Check sheet for the drawn part. Datum: minimum x, y, z corner. Units: mm. A direction names the side the tool comes from. Coordinates: 2 decimals unless noted, no trailing zeros. Write each loop counter-clockwise with the first axis right and the second up, starting at its lowest first coordinate (ties: lowest second). Pieces come first, ordered by that corner, then holes. Notation, with made-up numbers: M 58,-32.5 L 87,-32.5 A23 cw 87,-4.5 Z; hole C 5,56.25 d7. An arc over 180 degrees is marked long. Write item = value, one per line. Start each with the question number.
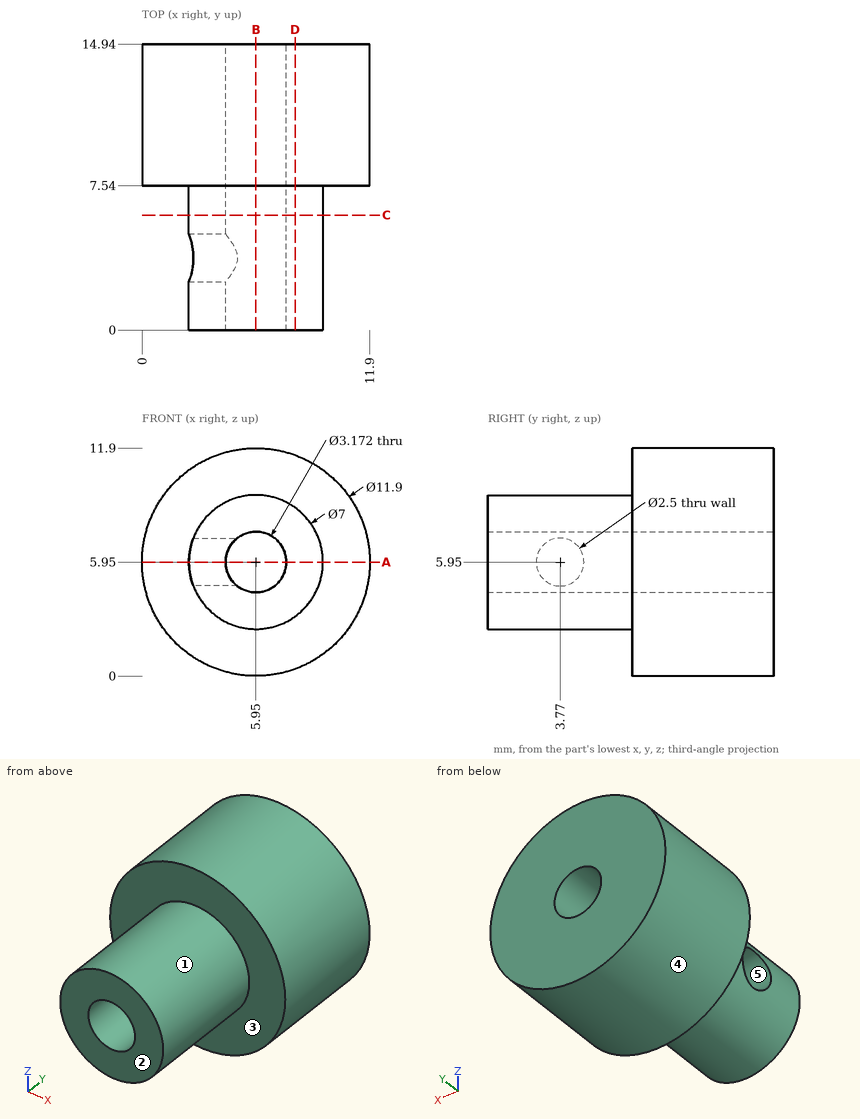
Q1. Gauge pin test, flat ends, axial feed: pin 1 (1.5 mm diameter, centred on x = 5, y = 5.5, fed in from -Z); pin 2 (4 mm diameter, centred on x = 2, y = 5.5, fed in from -Z); pin 3 (2 mm diameter, centred on y = 5, z = 8, fed in from -X). Record the tip position at first contact, or that the pin passes through.
Q2. Cross-section at C-C on y = 6. Enter the section's corners in (x, z).
Q3. Cross-section at D-D on x = 8. Enter the section's corners in (y, z).
Q4. Set-up check for the marked faces 1 and 2: record each of +Z, -Z, +X, -X, +Y, -Y from which the full face is reachable in a straight line by a thin tool's end or side.
Q5. Cross-section at A-A on z = 5.95. Enter the section's corners in (x, y), and give its area (3 significant figures).
Q6. Draft check along Z on the marked faces 3, 4 and 5. Enter one of: pulls with the +Z half, pulls with the -Z half, needs draft (parallel to the pull), parting line crosses it, or undercut.
Q7. Scan lines: L1, parallel to X at y = 5.25, z = 5.95; L2, parallel to X at y = 9.5, z = 5.95; L3, parallel to Y at x = 4.75, z = 1.75. Record each from-to range of solid material in increasing order.
Q8. Cross-section at B-B on x = 5.95. Enter the section's corners in (y, z).
Values found:
q1.pin_1 = 2.46
q1.pin_2 = 3.04
q1.pin_3 = 2.61
q2.outline = C 5.95,5.95 d7; hole C 5.95,5.95 d3.17
q3.outline = M 0,3.11 L 7.54,3.11 L 7.54,0.36 L 14.94,0.36 L 14.94,11.54 L 7.54,11.54 L 7.54,8.79 L 0,8.79 Z
q4.face_1 = -Y
q4.face_2 = +Z, -Z, +X, -X, -Y
q5.outline = M 0,7.54 L 2.45,7.54 L 2.45,5.02 L 4.36,5.02 L 4.36,14.94 L 0,14.94 Z; M 2.45,0 L 4.36,0 L 4.36,2.52 L 2.45,2.52 Z; M 7.54,0 L 9.45,0 L 9.45,7.54 L 11.9,7.54 L 11.9,14.94 L 7.54,14.94 Z
q5.area = 88.7 mm²
q6.face_3 = needs draft
q6.face_4 = parting line crosses it
q6.face_5 = undercut
q7.L1 = 2.45 to 4.36, 7.54 to 9.45
q7.L2 = 0 to 4.36, 7.54 to 11.9
q7.L3 = 7.54 to 14.94
q8.outline = M 0,2.45 L 7.54,2.45 L 7.54,0 L 14.94,0 L 14.94,4.36 L 0,4.36 Z; M 0,7.54 L 14.94,7.54 L 14.94,11.9 L 7.54,11.9 L 7.54,9.45 L 0,9.45 Z
